Could you check a few things on this model? Use its own coordinates, in mm. Face numbers are marked on the shaded views. A direction names the side the tool comes from. Give positions to 0.01 mm unless a question says otherwise; leave off trailing zeros. Order: outer loops, then holes, each group sorted by start corner. A loop starts at its lowest first (then second) coordinate and runs counter-clockwise, first axis right, second up. Notation, with made-up numbers: M 52,32 L 76,32 A23 cw 76,43 Z; hole C -36,25 d11. An arc over 180 degrees is marked long. Use a Markdown table: item, result. Add a question column.
```python
from build123d import *

# Parameters (mm, degrees)
SKETCH1_R           = 8
BOSS_EXTRUDE2_DEPTH = 30
SKETCH2_R           = 5
BOSS_EXTRUDE3_DEPTH = 40
SKETCH4_R           = 10.5
BOSS_EXTRUDE4_DEPTH = 40
SHELL1_T            = -1
CUT_EXTRUDE2_REACH  = 112.998
SKETCH5_R           = 9.5


with BuildPart() as part:
    # Sketch1 → Boss-Extrude2 (new body)
    with BuildSketch(Plane.XY):
        Circle(SKETCH1_R)
    extrude(amount=BOSS_EXTRUDE2_DEPTH)

    # Sketch2 → Boss-Extrude3 (add)
    with BuildSketch(Plane.XY.offset(30)):
        Circle(SKETCH2_R)
    extrude(amount=BOSS_EXTRUDE3_DEPTH)

    # Sketch4 → Boss-Extrude4 (add)
    with BuildSketch(Plane(origin=(0, 0, 0), x_dir=(-1, 0, 0), z_dir=(0, 0, -1))):
        Circle(SKETCH4_R)
    extrude(amount=BOSS_EXTRUDE4_DEPTH)

    # Shell1
    shell1_openings = [part.faces().sort_by_distance(p)[0] for p in [
        (0, 0, 70),
    ]]
    offset(amount=SHELL1_T, openings=shell1_openings, kind=Kind.INTERSECTION)

    # Sketch5 → Cut-Extrude2 (cut, up to next)
    with BuildSketch(Plane(origin=(0, 0, -40), x_dir=(-1, 0, 0), z_dir=(0, 0, -1)), mode=Mode.PRIVATE) as cut_extrude2_sk1:
        Circle(SKETCH5_R)
    cut_extrude2_tool1 = extrude(cut_extrude2_sk1.sketch, amount=-CUT_EXTRUDE2_REACH, mode=Mode.PRIVATE) & part.part
    add(cut_extrude2_tool1.solids().sort_by_distance((0, 0, -40))[0], mode=Mode.SUBTRACT)


solid = part.part
```
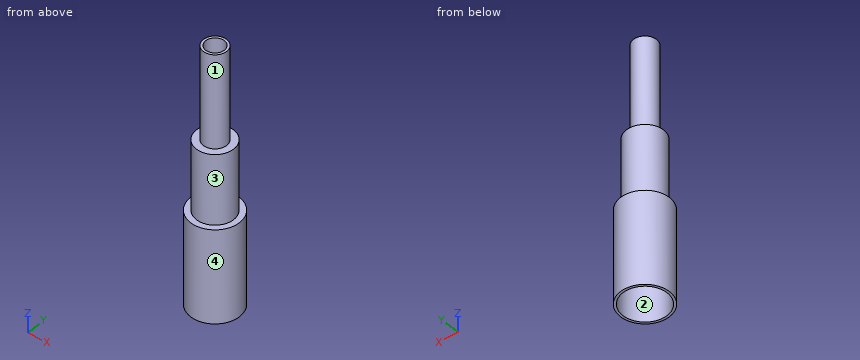
1) Suppose I cut it at D-D on z = -29. Please give me the cut outline in (x, y), and give its area (3 significant figures).
2) For the marked faces 3 and 4, which set-ups out of +Z, -Z, +X, -X, +Y, -Y let a thin tool reach every point of the face, with its end or its side?
3) Suppose I cut it at C-C on z = 45. Please give me the cut outline in (x, y).
4) Please list where these lines run through material, in increasing order: line 1 (Y direction, x = 0, z = -16); line 2 (Y direction, x = 0, z = 16.25); line 3 (X direction, y = 0.25, z = 39). Write a range as from..to.
5) For pin 1 (8 mm diameter, centred on y = 2.5, z = -4, fed in from +X); pin 2 (12.5 mm diameter, centred on x = 0, y = 0, fed in from -Z); pin 3 (3 mm diameter, centred on x = 1.5, z = 45, fed in from -Y); pin 4 (7 mm diameter, centred on x = 0, y = 0, fed in from +Z), each with a flat end and sliding along its axis, tell me the tip position at first contact or that it passes through.
6) We'd pull the mould along Y, two halves only. Please class the marked faces 1 and 2: pulls with the +Y half, pulls with the -Y half, needs draft (parallel to the pull), parting line crosses it, or undercut.
7) Suppose I cut it at A-A on y = 0. Please give me the cut outline in (x, z).
Values found:
| question | item | result |
|---|---|---|
| 1 | outline | C 0,0 d21; hole C 0,0 d19 |
| 1 | area | 62.8 mm^2 |
| 2 | face 3 | +Z |
| 2 | face 4 | +Z, -Z |
| 3 | outline | C 0,0 d10; hole C 0,0 d8 |
| 4 | line 1 | y = -10.5..-9.5, 9.5..10.5 |
| 4 | line 2 | y = -8..-7, 7..8 |
| 4 | line 3 | x = -4.99..-3.99, 3.99..4.99 |
| 5 | pin 1 | stops at x = 10.5 |
| 5 | pin 2 | stops at z = 29 |
| 5 | pin 3 | stops at y = -5 |
| 5 | pin 4 | passes through |
| 6 | face 1 | parting line crosses it |
| 6 | face 2 | undercut |
| 7 | outline | M -10.5,-40 L -9.5,-40 L -9.5,-1 L -7,-1 L -7,29 L -4,29 L -4,70 L -5,70 L -5,30 L -8,30 L -8,0 L -10.5,0 Z; M 4,29 L 7,29 L 7,-1 L 9.5,-1 L 9.5,-40 L 10.5,-40 L 10.5,0 L 8,0 L 8,30 L 5,30 L 5,70 L 4,70 Z |
